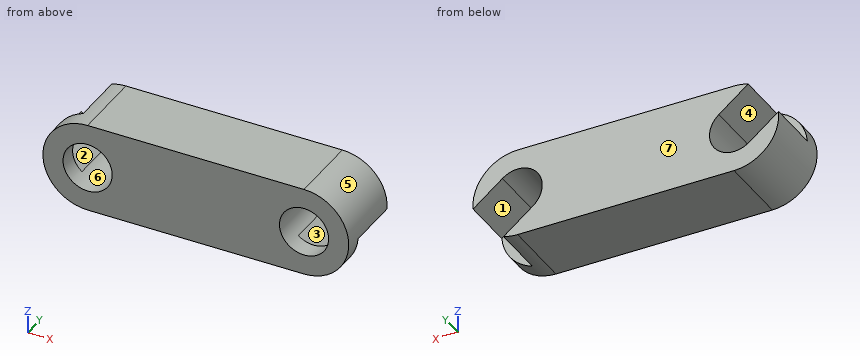
from build123d import *

# Parameters (mm, degrees)
SKETCH1_R           = 2.75
BOSS_EXTRUDE1_DEPTH = 8
CUT_EXTRUDE1_DEPTH  = 6


with BuildPart() as part:
    # Sketch1 → Boss-Extrude1 (new body)
    with BuildSketch(Plane(origin=(0, 0, 0), x_dir=(1, 0, 0), z_dir=(0, 1, 0))):
        with BuildLine():
            Line((-7.712527276, 6.5), (16.494909594, 6.5))
            ThreePointArc((16.494909594, 6.5), (21.494909594, 1.5), (16.494909594, -3.5))
            Line((16.494909594, -3.5), (-7.712527276, -3.5))
            ThreePointArc((-7.712527276, -3.5), (-12.712527276, 1.5), (-7.712527276, 6.5))
        make_face()
        with Locations(Location((-7.712527276, 1.5, 0), (0, 0, 270))):
            Circle(SKETCH1_R, mode=Mode.SUBTRACT)
        with Locations(Location((16.494909594, 1.5, 0), (0, 0, 270))):
            Circle(SKETCH1_R, mode=Mode.SUBTRACT)
    extrude(amount=BOSS_EXTRUDE1_DEPTH)

    # Sketch2 → Cut-Extrude1 (cut)
    with BuildSketch(Plane(origin=(0, 8, 0), x_dir=(1, 0, 0), z_dir=(0, 1, 0))):
        Polygon((14.7908878, 3.658427605), (18.198931387, -0.658427605), (28.129781504, 7.181717223), (24.721737917, 11.498572433), align=None)
        Polygon((-6.008505483, -0.658427605), (-9.41654907, 3.658427605), (-19.347399186, -4.181717223), (-15.939355599, -8.498572433), align=None)
    extrude(amount=-CUT_EXTRUDE1_DEPTH, mode=Mode.SUBTRACT)


solid = part.part
Geometry check sheet. Reference: the model listing, model coordinates, mm. Face numbers are marked on the shaded views. A direction names the side the tool comes from. Round coordinates to 2 decimals unless told otherwise and drop trailing zeros. Loops run counter-clockwise (first coordinate to the right, second up) from the corner with the lowest first, then second, coordinate; pieces in that order, holes last. Notation, with made-up numbers: (63.25, 39) - (85.25, 39) arc R28 cw to (85.25, 65) - close; hole circle Ø9 at (19.25, 30.25). An arc over 180 degrees is marked (long way). Answer as CSV lines item,"result".
(1) Release check for a two-part mould opening along Z. For the marked faces 5, 6 and 7 record: released by +Z, released by -Z, zero draft, split by the parting line, or undercut.
Output values:
face 5,"split by the parting line"
face 6,"undercut"
face 7,"zero draft"
(2) Cross-section at B-B, the plane y = 1.5. Enter the section's corners in (x, z).
Output values:
outline,"(-7.71, -6.5) - (16.49, -6.5) arc R5 ccw to (16.49, 3.5) - (-7.71, 3.5) arc R5 ccw to start; hole circle Ø5.5 at (-7.71, -1.5); hole circle Ø5.5 at (16.49, -1.5)"
(3) Cross-section at D-D, the plane z = 2.75. Enter the section's corners in (x, y), and give its area (3 significant figures).
Output values:
outline,"(-10.35, 0) - (19.13, 0) - (19.13, 8) - (-8.66, 8) - (-8.66, 2) - (-10.35, 2) - close"
area,"226 mm²"
(4) Cross-section at C-C, the plane z = -1.5. Enter the section's corners in (x, y), and give its area (3 significant figures).
Output values:
outline,"(-12.71, 0) - (-10.46, 0) - (-10.46, 2) - (-12.15, 2) - (-12.15, 8) - (-12.71, 8) - close; (-4.96, 0) - (13.74, 0) - (13.74, 8) - (-4.96, 8) - close; (19.24, 0) - (21.49, 0) - (21.49, 8) - (20.93, 8) - (20.93, 2) - (19.24, 2) - close"
area,"165 mm²"
(5) Cross-section at A-A, the plane z = 0.25. Enter the section's corners in (x, y), and give its area (3 significant figures).
Output values:
outline,"(-12.4, 0) - (-9.83, 0) - (-9.83, 2) - (-12.4, 2) - close; (-5.59, 0) - (14.37, 0) - (14.37, 8) - (-5.59, 8) - close; (18.62, 0) - (21.18, 0) - (21.18, 8) - (18.72, 8) - (18.72, 2) - (18.62, 2) - close"
area,"185 mm²"
(6) Material ranges on line 1 along X through (y, z) = (2.75, -1.5); line 2 along X through (y, z) = (1.25, -0.5); line 3 along Y through (x, z) = (20, -4.75), recorded low to high.
Output values:
line 1,"x = -12.71 to -12.15, -4.96 to 13.74, 20.93 to 21.49"
line 2,"x = -12.61 to -10.27, -5.15 to 13.93, 19.06 to 21.39"
line 3,"y = 0 to 2"
(7) Set-up check for the marked faces 1, 2, 3 and 4: record each of +Z, -Z, +X, -X, +Y, -Y from which the full face is reachable in a straight line by a thin tool's end or side.
Output values:
face 1,"-Z, +Y"
face 2,"+Z, +Y"
face 3,"+X, +Y"
face 4,"-X, +Y"
(8) Depth check by flat-ended pin: pin 1 Ø3.5 at (x, z) = (16.49, -1.5) entering from -Y; pin 2 Ø1 at (y, z) = (7, 0.5) entering from -X. Enter the tip coordinate at first touch or a pass-through.
Output values:
pin 1,"passes through"
pin 2,"stops at x = -6.44"
